Autodesk Inventor part; units mm, degrees
ref_plane "bolt2_to_body_XY" through (-10, 30.5, 0) normal (0, 1, 0) x (1, 0, 0)
ref_plane "bolt2_to_body_YZ" through (-10, 30.5, 0) normal (1, 0, 0) x (0, 0, -1)
ref_plane "bolt2_to_body_ZX" through (-10, 30.5, 0) normal (0, 0, -1) x (0, 1, 0)
sketch "Sketch_10" plane through (0, 0, 0) normal (0, 0, 1) x (1, 0, 0)
  line L0 (-16, 24) -> (-16, 0)
  line L1 (-16, 0) -> (16, 0)
  line L2 (16, 0) -> (16, 24)
  line L3 (16, 24) -> (4.899, 24)
  arc A0 (-4.899, 24) -> (4.899, 24) centre (0, 25) ccw
  line L4 (-4.899, 24) -> (-16, 24)
extrude "Extrusion1" add sketch "Sketch_10" along normal mid plane 12
sketch "Sketch2" plane through (4.899, 24, 6) normal (0, 1, 0) x (1, 0, 0)
  point P0 (5.101, 6)
hole "Hole1" at (10, 24, 0) direction (0, -1, 0) diameter 3.242 depth 6.0641 tip angle 120 countersink diameter 4 countersink angle 90
sketch "Sketch3" plane through (-16, 24, 6) normal (0, 1, 0) x (1, 0, 0)
  point P0 (6, 6)
hole "Hole2" at (-10, 24, 0) direction (0, -1, 0) diameter 3.242 depth 6.0641 tip angle 120 countersink diameter 4 countersink angle 90
sketch "Sketch_2" plane through (0, 0, 0) normal (0, 0, 1) x (1, 0, 0)
  circle A0 centre (10, 5) radius 2.25
extrude "Extrusion2" cut sketch "Sketch_2" along normal mid plane 12
sketch "Sketch_3" plane through (0, 0, 0) normal (0, 0, 1) x (1, 0, 0)
  circle A0 centre (-10, 5) radius 2.25
extrude "Extrusion3" cut sketch "Sketch_3" along normal mid plane 12
ref_plane "bolt2_to_body_XY" through (-10, 30.5, 0) normal (0, 1, 0) x (1, 0, 0)
ref_plane "bolt2_to_body_YZ" through (-10, 30.5, 0) normal (1, 0, 0) x (0, 0, -1)
ref_plane "bolt2_to_body_ZX" through (-10, 30.5, 0) normal (0, 0, -1) x (0, 1, 0)
ref_plane "bolt_to_body_XY" through (10, 30.5, 0) normal (0, 1, 0) x (1, 0, 0)
ref_plane "bolt_to_body_YZ" through (10, 30.5, 0) normal (1, 0, 0) x (0, 0, -1)
ref_plane "bolt_to_body_ZX" through (10, 30.5, 0) normal (0, 0, -1) x (0, 1, 0)
ref_plane "p_to_body_XY" through (0, 0, 0) normal (0, 1, 0) x (1, 0, 0)
ref_plane "p_to_body_YZ" through (0, 0, 0) normal (1, 0, 0) x (0, 0, -1)
ref_plane "p_to_body_ZX" through (0, 0, 0) normal (0, 0, -1) x (0, 1, 0)
properties part number "SHZA10-25_b"
Verification items for the finished model (mm, model axes). A direction names the side the tool comes from. Give positions to 0.01 mm unless a question says otherwise; leave off trailing zeros. Loops run counter-clockwise (first coordinate to the right, second up) from the corner with the lowest first, then second, coordinate; pieces in that order, holes last. Notation, with made-up numbers: (44.25, -17.75) - (84.25, -17.75) arc R27 cw to (84.25, 19.25) - close; hole circle Ø11 at (9.5, -3). An arc over 180 degrees is marked (long way). Write each question's results on one line, items separated by ' | '.
1) Sectioned sample at A-A on y = 5. Record the boundary of the cut face in (x, z), plus the area to 3 significant figures.
Solution:
outline: (-16, -6) - (-12.25, -6) - (-12.25, 6) - (-16, 6) - close; (-7.75, -6) - (7.75, -6) - (7.75, 6) - (-7.75, 6) - close; (12.25, -6) - (16, -6) - (16, 6) - (12.25, 6) - close | area: 276 mm2
2) Sectioned sample at D-D on x = -1.5. Record the boundary of the cut face in (y, z), plus the area to 3 significant figures.
Solution:
outline: (0, -6) - (20.23, -6) - (20.23, 6) - (0, 6) - close | area: 243 mm2
3) Sectioned sample at B-B on z = 3.75. Record the boundary of the cut face in (x, y).
Solution:
outline: (-16, 0) - (16, 0) - (16, 24) - (4.9, 24) arc R5 cw to (-4.9, 24) - (-16, 24) - close; hole circle Ø4.5 at (-10, 5); hole circle Ø4.5 at (10, 5)
4) Material ranges on L1, parallel to Z at x = 10, y = 20.55, recorded low to high. Write a range as from..to.
Solution:
L1: -6..-1.62, 1.62..6
5) Tool access check on faces 1 (the flat face through (0, 12, 6)), 2 (the cylindrical face through (-11.607, 20.739, -0.211)). Record the directions out of +Z, -Z, +X, -X, +Y, -Y that give a thin tool (end or side, any length) a straight path to the whole face; none if there is none.
Solution:
face 1: +Z, +X, -X, +Y, -Y | face 2: +Y
6) Depth check by flat-ended pin: P1, Ø1.5, axis at x = -8, z = 3.5, coming from the -Y side; P2, Ø3.5, axis at x = 10, z = 0, coming from the +Y side. Enter the tip coordinate at first touch or a pass-through.
Solution:
P1: y = 0 | P2: y = 23.75
7) Mould release check, pull along X, two halves, no side actions. Record for faces 3 (the flat face through (16, 12, 0)), 4 (the cylindrical face through (8.393, 20.739, -0.211)), 5 (the flat face through (-12, 24, -1)): pulls with the +X half, pulls with the -X half, needs draft (parallel to the pull), parting line crosses it, or undercut.
Solution:
face 3: pulls with the +X half | face 4: undercut | face 5: needs draft
8) Sectioned sample at C-C on x = 3.5. Record the boundary of the cut face in (y, z).
Solution:
outline: (0, -6) - (21.43, -6) - (21.43, 6) - (0, 6) - close
